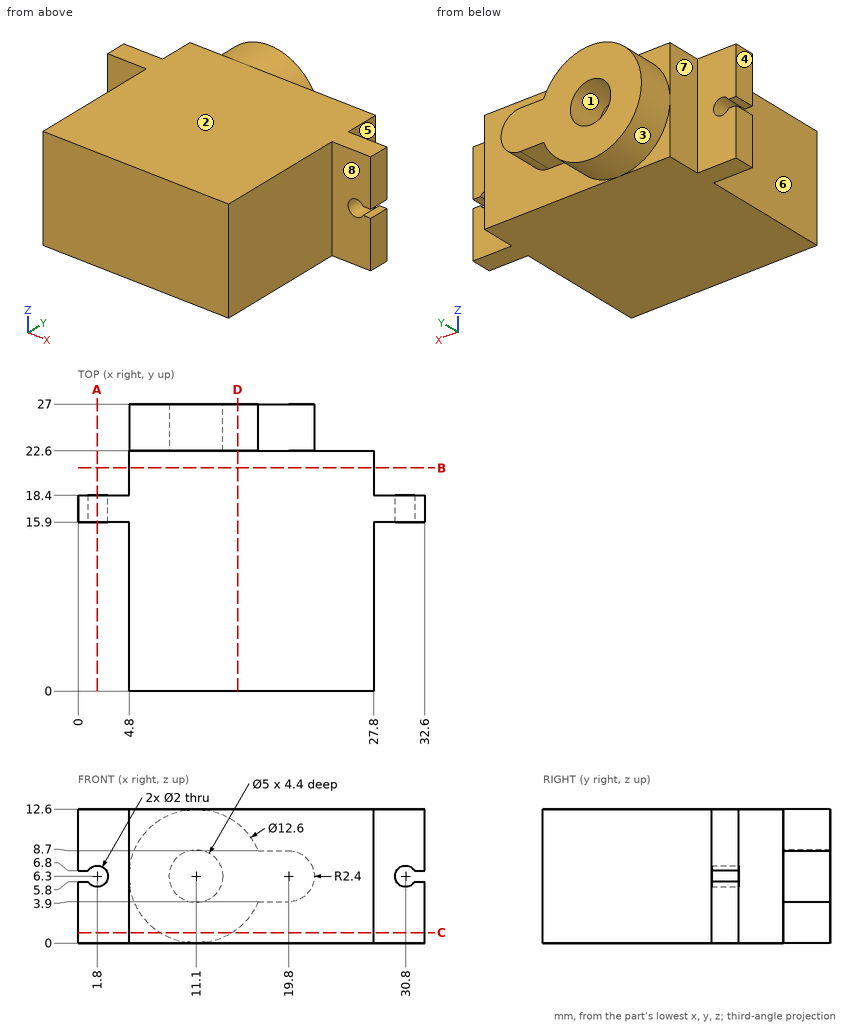
Study the drawing (mm; zero at the part's minimum x, y, z) and answer. A direction names the side the tool comes from. Coordinates: 2 decimals unless noted, no trailing zeros. Write each loop counter-clockwise with the first axis right and the second up, starting at its lowest first coordinate (ties: lowest second). Pieces come first, ordered by that corner, then holes. Notation, with made-up numbers: (-5.5, 5) - (38.5, 5) arc R19 ccw to (38.5, 33) - close; hole circle Ø2 at (0.5, 49.5). An arc over 180 degrees is marked (long way). Return JSON: item names as keys, results as strings. Group by question number.
1. Determine the mould class of the marked faces 1, 2, 3 and 4 for opening direction X: released by +X, released by -X, zero draft, split by the parting line, or undercut.
2. A cutting plane is placed at D-D, the plane x = 15. Determine the outline of the cut face in (y, z), plus the area to 3 significant figures.
3. Straight lines are drawn through the part: L1, parallel to X at y = 24.85, z = 6.3; L2, parallel to Z at x = 1.8, y = 17.4; L3, parallel to Z at x = 11.1, y = 25.45. For each, find the intervals that lie inside material, in ascending order.
4. A cutting plane is placed at A-A, the plane x = 1.8. Determine the outline of the cut face in (y, z), plus the area to 3 significant figures.
5. Which of the six approach directions +Z, -Z, +X, -X, +Y, -Y give full straight-line access (tool end or side, diameter ignored) to the marked faces 5, 6, 7 and 8?
6. A cutting plane is placed at B-B, the plane y = 21. Determine the outline of the cut face in (x, z), plus the area to 3 significant figures.
7. Given pin 1 (1.8 mm diameter, centred on x = 30.8, z = 6.3, fed in from +Y); pin 2 (1.4 mm diameter, centred on x = 1.5, z = 7, fed in from -Y); pin 3 (2.5 mm diameter, centred on x = 31, z = 4.5, fed in from +Y); pin 4 (3 mm diameter, centred on x = 11.1, z = 6.3, fed in from +Y), each flat-ended and moving along its own axis, determine where each tip first touches the part or whether it passes through.
8. A cutting plane is placed at C-C, the plane z = 1. Determine the outline of the cut face in (x, y), plus the area to 3 significant figures.
Ans:
{
 "1": {"face 1": "undercut", "face 2": "zero draft", "face 3": "split by the parting line", "face 4": "released by -X"},
 "2": {"outline": "(0, 0) - (22.6, 0) - (22.6, 1.35) - (27, 1.35) - (27, 11.25) - (22.6, 11.25) - (22.6, 12.6) - (0, 12.6) - close", "area": "328 mm²"},
 "3": {"L1": "4.8 to 8.6, 13.6 to 22.2", "L2": "0 to 5.3, 7.3 to 12.6", "L3": "0 to 3.8, 8.8 to 12.6"},
 "4": {"outline": "(15.9, 0) - (18.4, 0) - (18.4, 5.3) - (15.9, 5.3) - close; (15.9, 7.3) - (18.4, 7.3) - (18.4, 12.6) - (15.9, 12.6) - close", "area": "26.5 mm²"},
 "5": {"face 5": "+Z, -Z, +X, +Y", "face 6": "+Z, -Z, -X, -Y", "face 7": "+Z, -Z, -X, +Y", "face 8": "+Z, -Z, +X, -Y"},
 "6": {"outline": "(4.8, 0) - (27.8, 0) - (27.8, 12.6) - (4.8, 12.6) - close", "area": "290 mm²"},
 "7": {"pin 1": "through", "pin 2": "y = 15.9", "pin 3": "y = 18.4", "pin 4": "y = 22.6"},
 "8": {"outline": "(0, 15.9) - (4.8, 15.9) - (4.8, 0) - (27.8, 0) - (27.8, 15.9) - (32.6, 15.9) - (32.6, 18.4) - (27.8, 18.4) - (27.8, 22.6) - (14.51, 22.6) - (14.51, 27) - (7.69, 27) - (7.69, 22.6) - (4.8, 22.6) - (4.8, 18.4) - (0, 18.4) - close", "area": "574 mm²"}
}
